```python
from build123d import *

# Parameters (mm, degrees)
F1_DEPTH = 20
F3_DEPTH = 20


with BuildPart() as f1:
    # F0 (on Front) → F1 (new body)
    with BuildSketch(Plane.XZ):
        Polygon((-45, 34.875002), (-45, -30.124998), (0, -30.124998), (45, -30.124998), (45, 34.875002), (15, 34.875002), (15, 9.875002), (-15, 9.875002), (-15, 34.875002), align=None)
    extrude(amount=F1_DEPTH)

    # F2 (on face) → F3 (join)
    with BuildSketch(Plane.XZ.offset(20)):
        Polygon((-45, 34.875002), (-45, -30.124998), (-15, -30.124998), align=None)
        Polygon((45, 34.875002), (15, -30.124998), (45, -30.124998), align=None)
    extrude(amount=F3_DEPTH)


solid = f1.part
```
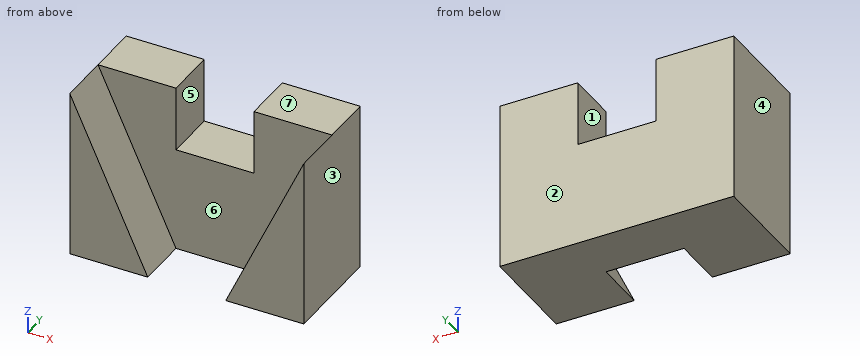
Input: part model. Units: mm. Frame: model coordinates. Face numbers are marked on the shaded views. A direction names the side the tool comes from. Give positions to 0.01 mm unless a question says otherwise; leave off trailing zeros. Order: outer loops, then holes, each group sorted by start corner. A loop starts at its lowest first (then second) coordinate and runs counter-clockwise, first axis right, second up. Notation, with made-up numbers: M 24.5,88.5 L 71.5,88.5 A20 ccw 71.5,108.5 Z; hole C -33,52.25 d11. An arc over 180 degrees is marked long. Return JSON: item names as keys, results as strings.
Item 1: First-contact query: P1, Ø1.5, axis at x = 0, z = 9, coming from the -Y side; P2, Ø22, axis at x = 0.5, y = -9.5, coming from the +Z side (3 decimals). Flat tips, straight axial feed; report the tip coordinate or a pass-through.
Solutions:
{"P1": "y = -20", "P2": "z = 9.875"}
Item 2: Access query for the marked faces 5, 6 and 7. Directions: +Z, -Z, +X, -X, +Y, -Y. A direction counts if a zero-diameter tool reaches every point of the face in a straight line with its end or side. Return the directions, or none.
Solutions:
{"face 5": "+Z, +Y, -Y", "face 6": "+Z, -Y", "face 7": "+Z, +X, -X, +Y, -Y"}
Item 3: Cut plane D-D (z = -2.5). Return loops of the section in (x, y), then the cut area to 3 significant figures.
Solutions:
{"outline": "M -45,-40 L -27.75,-40 L -27.75,-20 L 27.75,-20 L 27.75,-40 L 45,-40 L 45,0 L -45,0 Z", "area": "2,490 mm^2"}
Item 4: Pull-direction query (X, two-part tool) for the marked faces 1, 2, 3 and 4; classes: +X half, -X half, draft (parallel to the pull), parting line (faces both ways), or undercut.
Solutions:
{"face 1": "undercut", "face 2": "draft", "face 3": "+X half", "face 4": "-X half"}
Item 5: Cut plane A-A (z = 30). Return loops of the section in (x, y), then the cut area to 3 significant figures.
Solutions:
{"outline": "M -45,-40 L -42.75,-40 L -42.75,-20 L -15,-20 L -15,0 L -45,0 Z; M 15,-20 L 42.75,-20 L 42.75,-40 L 45,-40 L 45,0 L 15,0 Z", "area": "1,290 mm^2"}
Item 6: Cut plane B-B (y = -10.5). Return loops of the section in (x, z) (3 decimals).
Solutions:
{"outline": "M -45,-30.125 L 45,-30.125 L 45,34.875 L 15,34.875 L 15,9.875 L -15,9.875 L -15,34.875 L -45,34.875 Z"}
Item 7: Cut plane C-C (y = -30.5). Return loops of the section in (x, z) (3 decimals).
Solutions:
{"outline": "M -45,-30.125 L -15,-30.125 L -45,34.875 Z; M 15,-30.125 L 45,-30.125 L 45,34.875 Z"}
Item 8: Ray query, probe 1 along X at (y, z) = (-9, 28.5); probe 2 along Y at (x, z) = (-22.5, 13.5); probe 3 along X at (y, z) = (-31.5, 23.5). Return the intervals inside material, ascending.
Solutions:
{"probe 1": "-45 to -15, 15 to 45", "probe 2": "-20 to 0", "probe 3": "-45 to -39.75, 39.75 to 45"}
